The model under review builds one solid part; all positions refer to its coordinate system, in mm. A direction names the side the tool comes from. Coordinates: 2 decimals unless noted, no trailing zeros. Order: outer loops, then holes, each group sorted by start corner. A loop starts at its lowest first (then second) coordinate and runs counter-clockwise, first axis right, second up.
from build123d import *

# Parameters (mm, degrees)
CUT_EXTRUDE1_DEPTH      = 35.471002306
CUT_EXTRUDE1_DEPTH_BACK = 35.471002306
SKETCH2_W               = 6
SKETCH2_H               = 8
SKETCH3_R               = 2.5
CUT_EXTRUDE2_DEPTH      = 10
CHAMFER1_SIZE           = 0.3


with BuildPart() as part:
    # Sketch1 → Revolve1 (revolve)
    with BuildSketch(Plane(origin=(0, 0, 0), x_dir=(0, 0, -1), z_dir=(1, 0, 0)), mode=Mode.PRIVATE) as revolve1_sk:
        Polygon((17.5, 6), (-17.5, 6), (-17.5, 21), (-9.5, 21), (-9.5, 11), (17.5, 11), align=None)
    revolve(revolve1_sk.sketch.rotate(Axis((0, 0, 27), (0, 0, -1)), 90), axis=Axis((0, 0, 27), (0, 0, -1)))

    # Sketch2 → Cut-Extrude1 (cut, two sides: drawn at the far end of the back side and taken through both)
    with BuildSketch(Plane(origin=(0, 0, 0), x_dir=(1, 0, 0), z_dir=(0, 1, 0)).offset(-CUT_EXTRUDE1_DEPTH_BACK)):
        with Locations((-18, -13.5)):
            Rectangle(SKETCH2_W, SKETCH2_H)
        with Locations((18, -13.5)):
            Rectangle(SKETCH2_W, SKETCH2_H)
    extrude(amount=CUT_EXTRUDE1_DEPTH + CUT_EXTRUDE1_DEPTH_BACK, mode=Mode.SUBTRACT)

    # Sketch3 → Cut-Extrude2 (cut)
    with BuildSketch(Plane.XY.offset(17.5)):
        with Locations((0, 16)):
            Circle(SKETCH3_R)
        with Locations((11.313708499, 11.313708499)):
            Circle(SKETCH3_R)
        with Locations((11.313708499, -11.313708499)):
            Circle(SKETCH3_R)
        with Locations((0, -16)):
            Circle(SKETCH3_R)
        with Locations((-11.313708499, -11.313708499)):
            Circle(SKETCH3_R)
        with Locations((-11.313708499, 11.313708499)):
            Circle(SKETCH3_R)
    extrude(amount=-CUT_EXTRUDE2_DEPTH, mode=Mode.SUBTRACT)

    # Chamfer1
    chamfer1_edges = [part.edges().sort_by_distance(p)[0] for p in [
        (0, -21, 9.5),
        (-15, 0, 9.5),
        (0, -21, 17.5),
        (-15, 0, 17.5),
        (0, 21, 9.5),
        (15, 0, 9.5),
        (0, 21, 17.5),
        (15, 0, 17.5),
        (-11, 0, -17.5),
        (-11, 0, 9.5),
        (-2.5, 16, 9.5),
        (-2.5, 16, 17.5),
        (8.813708499, 11.313708499, 9.5),
        (-6, 0, 17.5),
        (8.813708499, 11.313708499, 17.5),
        (8.813708499, -11.313708499, 9.5),
        (8.813708499, -11.313708499, 17.5),
        (-2.5, -16, 9.5),
        (-6, 0, -17.5),
        (-2.5, -16, 17.5),
        (-13.813708499, -11.313708499, 9.5),
        (-13.813708499, -11.313708499, 17.5),
        (-13.813708499, 11.313708499, 9.5),
        (-13.813708499, 11.313708499, 17.5),
    ]]
    chamfer(chamfer1_edges, length=CHAMFER1_SIZE)


solid = part.part
(1) Consider section B-B (x = 0). Give the number of separate pieces and of enclosed holes in the cut face, then the cut area to 3 significant figures.
(2) Consider section A-A (y = 0). Give the boundary of the cut face in (x, z), then the cut area to 3 significant figures.
(3) Wall thickness on line 1 (Y direction, x = -1.5, z = 13); line 2 (Z direction, x = -12, y = -5); line 3 (Y direction, x = 9.5, z = 10): over which ranges is each line inside the solid? List them lowest first.
(4) Tool access review of faces 1 (the face through (-6.7, -9.5, 9.5)), 2 (the face through (5.723, -1.802, 0.241)): name each direction out of +Z, -Z, +X, -X, +Y, -Y from which nothing blocks a thin tool from reaching the whole face with its end or side.
(5) Insertion check: pin 1 Ø12 at (x, y) = (10.5, -16) entering from -Z; pin 2 Ø11 at (x, y) = (0, 0) entering from -Z; pin 3 Ø5 at (y, z) = (-0.5, 1.5) entering from +X; pin 4 Ø3 at (y, z) = (-8.5, 2) entering from +X. Each pin has a flat end and moves straight along its axis. Give the tip position at first contact, or say it passes through.
(6) The part is to be moulded in two halves that separate along Y. For faces 3 (the face through (-0.23, 20.81, 9.61)), 4 (the face through (15, 0, 14)), 5 (the face through (-0.54, 13.56, 13.55)), say which applies: +Y half, -Y half, draft (parallel to the pull), parting line (faces both ways), or undercut.
Findings:
1. separate pieces: 4
1. enclosed holes: 0
1. area: 429 mm2
2. outline: (-15, 9.8) - (-14.7, 9.5) - (-11.3, 9.5) - (-11, 9.2) - (-11, -17.2) - (-10.7, -17.5) - (-6.3, -17.5) - (-6, -17.2) - (-6, 17.2) - (-6.3, 17.5) - (-14.7, 17.5) - (-15, 17.2) - close; (6, -17.2) - (6.3, -17.5) - (10.7, -17.5) - (11, -17.2) - (11, 9.2) - (11.3, 9.5) - (14.7, 9.5) - (15, 9.8) - (15, 17.2) - (14.7, 17.5) - (6.3, 17.5) - (6, 17.2) - close
2. area: 414 mm2
3. line 1: y = -20.95 to -18, -14 to -5.81, 5.81 to 14, 18 to 20.95
3. line 2: z = 9.5 to 17.5
3. line 3: y = -18.73 to -13.03, -9.59 to 9.59, 13.03 to 18.73
4. face 1: -Z
4. face 2: +Z, -Z
5. pin 1: stops at z = 9.5
5. pin 2: passes through
5. pin 3: stops at x = 11
5. pin 4: stops at x = 8.49
6. face 3: +Y half
6. face 4: draft
6. face 5: undercut
